from build123d import *

# Parameters (mm, degrees)
ESBO_O1_W                = 30
ESBO_O1_H                = 10
ESBO_O1_W_2              = 26
ESBO_O1_H_2              = 6
RESSALTO_EXTRUS_O1_DEPTH = 80
ESBO_O2_R                = 4
CORTE_EXTRUS_O1_DEPTH    = 10
ESBO_O4_R                = 1.5
CORTE_EXTRUS_O2_DEPTH    = 2
ESBO_O6_R                = 2
CORTE_EXTRUS_O4_DEPTH    = 2
ESBO_O7_W                = 26
ESBO_O7_H                = 6
CORTE_EXTRUS_O5_DEPTH    = 2
ESBO_O8_W                = 26
ESBO_O8_H                = 6
CORTE_EXTRUS_O6_DEPTH    = 2
ESBO_O10_W               = 26
ESBO_O10_H               = 8
CORTE_EXTRUS_O7_DEPTH    = 2


with BuildPart() as part:
    # Esboço1 → Ressalto-extrusão1 (new body)
    with BuildSketch(Plane.XY):
        Rectangle(ESBO_O1_W, ESBO_O1_H)
        Rectangle(ESBO_O1_W_2, ESBO_O1_H_2, mode=Mode.SUBTRACT)
    extrude(amount=RESSALTO_EXTRUS_O1_DEPTH)

    # Esboço2 → Corte-extrusão1 (cut)
    with BuildSketch(Plane(origin=(0, 5, 0), x_dir=(1, 0, 0), z_dir=(0, 1, 0))):
        with Locations(Location((0, -40, 0), (0, 0, 270))):
            Circle(ESBO_O2_R)
    extrude(amount=-CORTE_EXTRUS_O1_DEPTH, mode=Mode.SUBTRACT)

    # Esboço4 → Corte-extrusão2 (cut)
    with BuildSketch(Plane(origin=(0, 5, 0), x_dir=(1, 0, 0), z_dir=(0, 1, 0))):
        with Locations(Location((0, -31, 0), (0, 0, 270))):
            Circle(ESBO_O4_R)
        with Locations(Location((7.794228634, -44.5, 0), (0, 0, 270))):
            Circle(ESBO_O4_R)
        with Locations(Location((-7.794228634, -44.5, 0), (0, 0, 270))):
            Circle(ESBO_O4_R)
    extrude(amount=-CORTE_EXTRUS_O2_DEPTH, mode=Mode.SUBTRACT)

    # Esboço6 → Corte-extrusão4 (cut)
    with BuildSketch(Plane(origin=(0, -5, 0), x_dir=(-1, 0, 0), z_dir=(0, -1, 0))):
        with Locations(Location((0, -56, 0), (0, 0, 90))):
            Circle(ESBO_O6_R)
    corte_extrus_o4 = extrude(amount=-CORTE_EXTRUS_O4_DEPTH, mode=Mode.SUBTRACT)

    # Espelhar1: Corte-extrusão4 across plane
    add(corte_extrus_o4.mirror(Plane.XY.offset(40)), mode=Mode.SUBTRACT)

    # Esboço7 → Corte-extrusão5 (cut)
    with BuildSketch(Plane(origin=(0, 5, 0), x_dir=(1, 0, 0), z_dir=(0, 1, 0))):
        with Locations((0, -24)):
            Rectangle(ESBO_O7_W, ESBO_O7_H)
    corte_extrus_o5 = extrude(amount=-CORTE_EXTRUS_O5_DEPTH, mode=Mode.SUBTRACT)

    # Espelhar2: Corte-extrusão5 across plane
    add(corte_extrus_o5.mirror(Plane.XY.offset(40)), mode=Mode.SUBTRACT)

    # Esboço8 → Corte-extrusão6 (cut)
    with BuildSketch(Plane(origin=(0, -5, 0), x_dir=(-1, 0, 0), z_dir=(0, -1, 0))):
        with Locations((0, -31)):
            Rectangle(ESBO_O8_W, ESBO_O8_H)
    extrude(amount=-CORTE_EXTRUS_O6_DEPTH, mode=Mode.SUBTRACT)

    # Esboço10 → Corte-extrusão7 (cut)
    with BuildSketch(Plane(origin=(0, -5, 0), x_dir=(-1, 0, 0), z_dir=(0, -1, 0))):
        with Locations((0, -44)):
            Rectangle(ESBO_O10_W, ESBO_O10_H)
    extrude(amount=-CORTE_EXTRUS_O7_DEPTH, mode=Mode.SUBTRACT)


solid = part.part
Geometry: final body of the model. Coordinates: model frame, mm. A direction names the side the tool comes from. Coordinates: 2 decimals unless noted, no trailing zeros. Order: outer loops, then holes, each group sorted by start corner. A loop starts at its lowest first (then second) coordinate and runs counter-clockwise, first axis right, second up. Notation, with made-up numbers: (45.5, 82.25) - (102.5, 82.25) arc R17 cw to (102.5, 99.25) - close; hole circle Ø11 at (16.5, 78.5). An arc over 180 degrees is marked (long way). Use one line per item in the form item = value.
1) Section A-A (z = 56). Return loops of the section in (x, y).
Solutions:
outline = (-15, -5) - (-2, -5) - (-2, -3) - (-13, -3) - (-13, 5) - (-15, 5) - close; (2, -5) - (15, -5) - (15, 5) - (13, 5) - (13, -3) - (2, -3) - close
2) Section C-C (y = 0.25). Return loops of the section in (x, z), then the cut area to 3 significant figures.
Solutions:
outline = (-15, 0) - (-13, 0) - (-13, 80) - (-15, 80) - close; (13, 0) - (15, 0) - (15, 80) - (13, 80) - close
area = 320 mm^2
3) Section B-B (x = -5.5). Return loops of the section in (y, z), then the cut area to 3 significant figures.
Solutions:
outline = (-5, 0) - (-3, 0) - (-3, 28) - (-5, 28) - close; (-5, 34) - (-3, 34) - (-3, 40) - (-5, 40) - close; (-5, 48) - (-3, 48) - (-3, 80) - (-5, 80) - close; (3, 0) - (5, 0) - (5, 21) - (3, 21) - close; (3, 27) - (5, 27) - (5, 53) - (3, 53) - close; (3, 59) - (5, 59) - (5, 80) - (3, 80) - close
area = 268 mm^2
4) Section D-D (y = -4.25). Return loops of the section in (x, z), then the cut area to 3 significant figures.
Solutions:
outline = (-15, 0) - (15, 0) - (15, 80) - (-15, 80) - close; hole (-13, 28) - (13, 28) - (13, 34) - (-13, 34) - close; hole (-13, 40) - (-4, 40) arc R4 ccw to (4, 40) - (13, 40) - (13, 48) - (-13, 48) - close; hole circle Ø4 at (0, 24); hole circle Ø4 at (0, 56)
area = 1,990 mm^2
5) Set-up query: faces 4 (the face through (0, -4, 36)), 5 (the face through (0, -4, 28)), 6 (the face through (0, 4, 21)), 7 (the face through (0, -3, 64)). Return all of +Z, -Z, +X, -X, +Y, -Y with unobstructed straight access to the full face (end or side cutting, diameter ignored); none if empty.
Solutions:
face_4 = +Y, -Y
face_5 = -Y
face_6 = +Y
face_7 = +Z, -Z
6) Pin query (flat end, axial travel): pin 1 (5 mm diameter, centred on x = -6.5, z = 43, fed in from -Y). Return the tip coordinate at first contact, or that it passes through.
Solutions:
pin_1 = 3
7) Mould query, pull axis Z, two halves, no side actions, for faces 1 (the face through (0, 3, 69)), 2 (the face through (0.07, 4.01, 29.5)), 3 (the face through (-0.2, 3.4, 0)). Classes: +Z half, -Z half, draft (parallel to the pull), parting line (faces both ways), or undercut.
Solutions:
face_1 = draft
face_2 = undercut
face_3 = -Z half
8) Ray query, L1, parallel to X at y = -0.5, z = 75.5; L2, parallel to Z at x = -5, y = 3.5; L3, parallel to Y at x = -11.5, z = 4.5. Return the intervals inside material, ascending.
Solutions:
L1 = -15 to -13, 13 to 15
L2 = 0 to 21, 27 to 53, 59 to 80
L3 = -5 to -3, 3 to 5
